Print and shaded views of the part. All mm, measured from the part's lowest x, y and z. Round coordinates to 2 decimals unless told otherwise and drop trailing zeros. Order: outer loops, then holes, each group sorted by start corner. A loop starts at its lowest first (then second) coordinate and runs counter-clockwise, first axis right, second up.
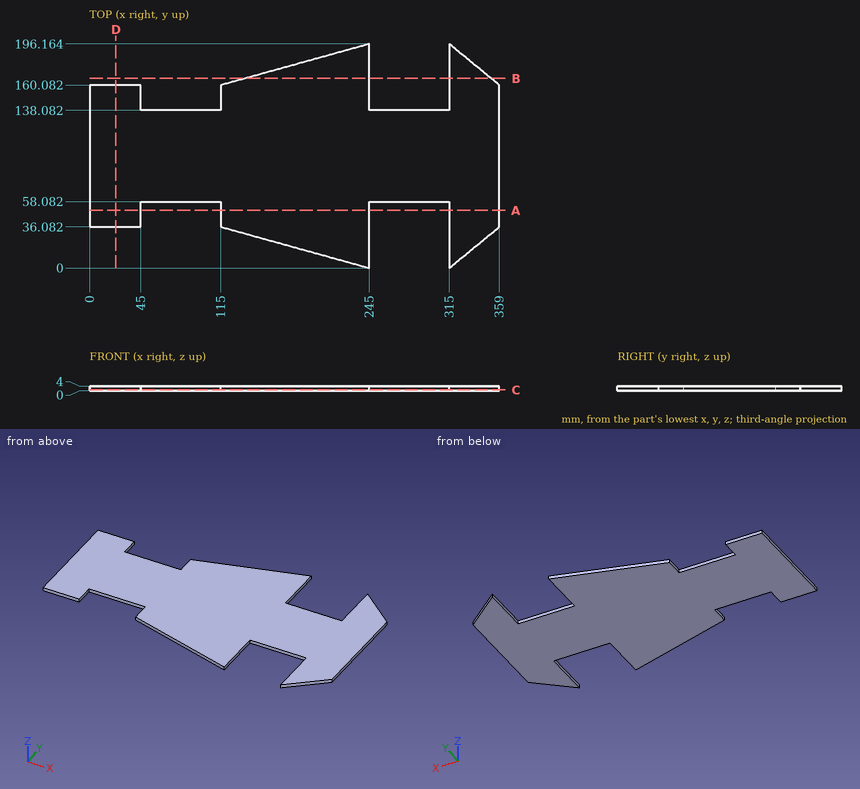
1. Cut at A-A, the plane y = 50.5. Write the cut outline in (x, z).
2. Cut at D-D, the plane x = 23. Write the cut outline in (y, z).
3. Pin check, flat tips, straight feed: P1, Ø2, axis at x = 27.5, z = 2.5, coming from the -Y side; P2, Ø2, axis at x = 94, z = 1.5, coming from the -Y side; P3, Ø2, axis at x = 79.5, z = 2.5, coming from the +Y side. Stop position of each tip, or through.
4. Drill centre lines: line 1 (X direction, y = 148.5, z = 1.35); line 2 (Y direction, x = 21.5, z = 1.4); line 3 (Y direction, x = 275, z = 1.45). Where is each one in solid material? Low to high.
5. Cut at C-C, the plane z = 0.6. Write the cut outline in (x, y).
6. Cut at B-B, the plane y = 166. Write the cut outline in (x, z).
Outcome:
1. outline: (0, 0) - (45, 0) - (45, 4) - (0, 4) - close; (115, 0) - (245, 0) - (245, 4) - (115, 4) - close; (315, 0) - (359, 0) - (359, 4) - (315, 4) - close
2. outline: (36.08, 0) - (160.08, 0) - (160.08, 4) - (36.08, 4) - close
3. P1: stops at y = 36.08
3. P2: stops at y = 58.08
3. P3: stops at y = 138.08
4. line 1: x = 0 to 45, 115 to 245, 315 to 359
4. line 2: y = 36.08 to 160.08
4. line 3: y = 58.08 to 138.08
5. outline: (0, 36.08) - (45, 36.08) - (45, 58.08) - (115, 58.08) - (115, 36.08) - (245, 0) - (245, 58.08) - (315, 58.08) - (315, 0) - (359, 36.08) - (359, 160.08) - (315, 196.16) - (315, 138.08) - (245, 138.08) - (245, 196.16) - (115, 160.08) - (115, 138.08) - (45, 138.08) - (45, 160.08) - (0, 160.08) - close
6. outline: (136.32, 0) - (245, 0) - (245, 4) - (136.32, 4) - close; (315, 0) - (351.78, 0) - (351.78, 4) - (315, 4) - close
